Could you check a few things on this model? Use its own coordinates, in mm. A direction names the side the tool comes from. Round coordinates to 2 decimals unless told otherwise and drop trailing zeros. Write each loop counter-clockwise with the first axis right and the second up, starting at its lowest first coordinate (ties: lowest second). Pieces come first, ordered by that corner, then holes. Notation, with made-up numbers: (-34, 64) -> (17, 64) arc R18 cw to (17, 93) -> close; hole circle Ø3 at (-12, 5). An arc over 180 degrees is marked (long way). Return JSON: item names as keys, results as strings.
from build123d import *

# Parameters (mm, degrees)
F1_DEPTH = 6.35
F3_DEPTH = 12.701
F6_R     = 2.54
F7_SIZE  = 2.54


with BuildPart() as f1:
    # F0 (on Top) → F1 (new body, symmetric)
    with BuildSketch(Plane.XY):
        with BuildLine():
            Line((21.59, 7.62), (-21.59, 7.62))
            ThreePointArc((-21.59, 7.62), (-44.45, 0), (-21.59, -7.62))
            Line((-21.59, -7.62), (21.59, -7.62))
            ThreePointArc((21.59, -7.62), (44.45, 0), (21.59, 7.62))
        make_face()
    extrude(amount=F1_DEPTH, both=True)

    # F4: F3 across plane


with BuildPart() as f3:
    # F2 (on face) → F3 (new body, through all)
    with BuildSketch(Plane(origin=(0, 0, -6.35), x_dir=(1, 0, 0), z_dir=(0, 0, -1))):
        Polygon((-43.632001, 9.581707), (-49.164003, 0), (-43.632001, -9.581707), (-32.567999, -9.581707), (-27.035997, 0), (-32.567999, 9.581707), align=None)
    extrude(amount=-F3_DEPTH)


with BuildPart() as f1_1:
    add(f1.part)
    add(f3.part.mirror(Plane.YZ), mode=Mode.SUBTRACT)

    # F5: cut F3
    add(f3.part, mode=Mode.SUBTRACT)

    # F6
    f6_edges = [f1_1.edges().sort_by_distance(p)[0] for p in [
        (0, -7.62, 6.35),
        (-30.410502, 12.629162, 6.35),
        (-30.410502, -12.629162, 6.35),
        (0, 7.62, 6.35),
        (30.410502, -12.629162, 6.35),
        (30.410502, 12.629162, 6.35),
    ]]
    fillet(f6_edges, radius=F6_R)

    # F7
    f7_edges = [f1_1.edges().sort_by_distance(p)[0] for p in [
        (30.410502, -12.629162, -6.35),
        (30.410502, 12.629162, -6.35),
        (0, -7.62, -6.35),
        (0, 7.62, -6.35),
        (-30.410502, 12.629162, -6.35),
        (-30.410502, -12.629162, -6.35),
    ]]
    chamfer(f7_edges, length=F7_SIZE)


solid = f1_1.part
1) I want a section at A-A, the plane x = 19. Please give me the cut outline in (y, z).
Return value:
{"outline": "(-7.62, -3.81) -> (-5.08, -6.35) -> (5.08, -6.35) -> (7.62, -3.81) -> (7.62, 3.81) arc R2.54 ccw to (5.08, 6.35) -> (-5.08, 6.35) arc R2.54 ccw to (-7.62, 3.81) -> close"}
2) For faces 1 (the face through (0, 7.62, 0)), 2 (the face through (-0.321, 6.896, 5.586)), 3 (the face through (-36, -9.582, 0)), which set-ups out of +Z, -Z, +X, -X, +Y, -Y let a thin tool reach every point of the face, with its end or its side?
Return value:
{"face 1": "+Z, -Z, +Y", "face 2": "+Z, +Y", "face 3": "+Z, -Z, -X"}
3) I want a section at B-B, the plane z = -2.5. Please give me the cut outline in (x, y), and give its area (3 significant figures).
Return value:
{"outline": "(-40.09, -9.58) arc R12.7 ccw to (-21.59, -7.62) -> (21.59, -7.62) arc R12.7 ccw to (40.09, -9.58) -> (32.57, -9.58) -> (27.04, 0) -> (32.57, 9.58) -> (40.09, 9.58) arc R12.7 ccw to (21.59, 7.62) -> (-21.59, 7.62) arc R12.7 ccw to (-40.09, 9.58) -> (-32.57, 9.58) -> (-27.04, 0) -> (-32.57, -9.58) -> close", "area": "1,110 mm²"}
4) Thinking about a two-plate mould opening in X: for faces 4 (the face through (-0.32, -6.37, -5.06)), 5 (the face through (29.84, 4.86, -0.09)), 6 (the face through (36, -9.582, 0)), 7 (the face through (0, -7.62, 0)), which applies, pulls with the +X half, pulls with the -X half, needs draft (parallel to the pull), parting line crosses it, or undercut?
Return value:
{"face 4": "undercut", "face 5": "pulls with the +X half", "face 6": "needs draft", "face 7": "undercut"}
5) I want a section at D-D, the plane z = 4.5. Please give me the cut outline in (x, y).
Return value:
{"outline": "(-39.94, -9.58) arc R12.6 ccw to (-21.64, -7.52) -> (21.64, -7.52) arc R12.6 ccw to (39.94, -9.58) -> (32.57, -9.58) -> (27.04, 0) -> (32.57, 9.58) -> (39.94, 9.58) arc R12.6 ccw to (21.64, 7.52) -> (-21.64, 7.52) arc R12.6 ccw to (-39.94, 9.58) -> (-32.57, 9.58) -> (-27.04, 0) -> (-32.57, -9.58) -> close"}
6) Will these pins go through, and if not, where does the flat tip stop? pin 1 Ø5 at (y, z) = (-6, 2.5) entering from +X; pin 2 Ø4 at (y, z) = (0.5, 0.5) entering from +X; pin 3 Ø6 at (x, z) = (37.5, 2.5) entering from +Y.
Return value:
{"pin 1": "x = 31.94", "pin 2": "x = 28.48", "pin 3": "y = 12.4"}
7) I want a section at C-C, the plane y = -2.75. Please give me the cut outline in (x, z).
Return value:
{"outline": "(-28.62, -6.35) -> (28.62, -6.35) -> (28.62, 6.35) -> (-28.62, 6.35) -> close"}
8) If I drill on probe 1 along Y at (x, z) = (-9, 3.25); probe 2 along X at (y, z) = (-8, 2.25); probe 3 along X at (y, z) = (-9.75, -3), over which ranges is the centre line in solid material (lowest first)? Write a range as [from, to].
Return value:
{"probe 1": "[-7.62, 7.62]", "probe 2": "[-31.65, -21.89], [21.89, 31.65]", "probe 3": "[-39.89, -23.61], [23.61, 39.89]"}
